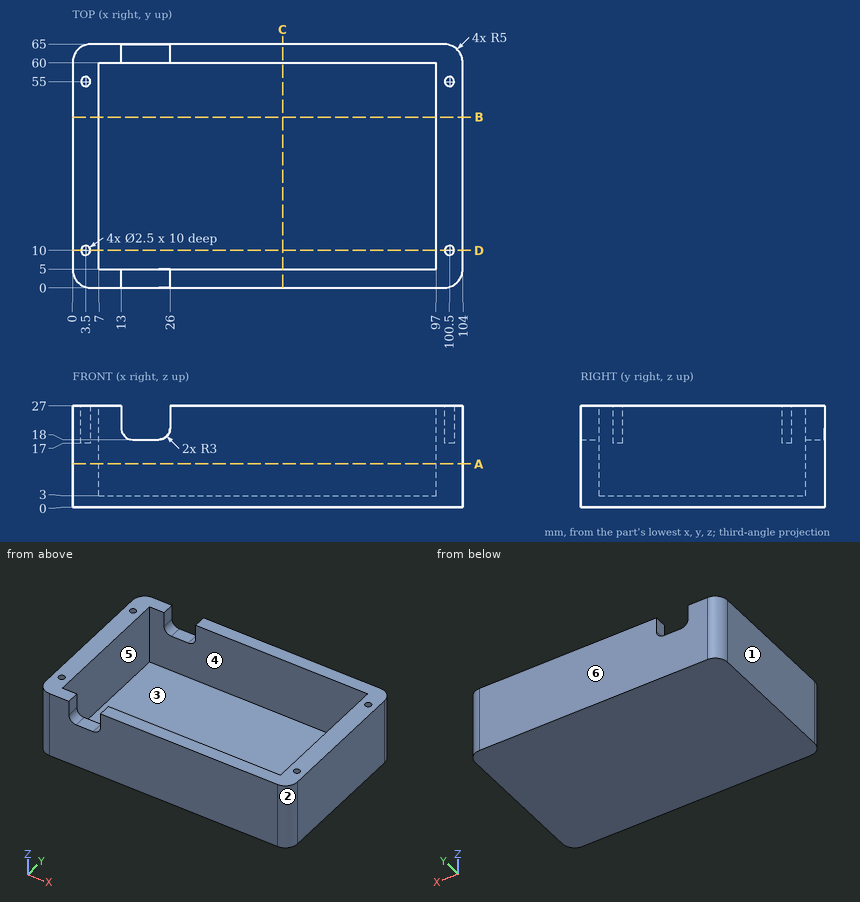
Study the drawing (mm; zero at the part's minimum x, y, z) and answer. A direction names the side the tool comes from. Round coordinates to 2 decimals unless told otherwise and drop trailing zeros. Write each loop counter-clockwise with the first axis right and the second up, starting at its lowest first coordinate (ties: lowest second). Pieces come first, ordered by that corner, then holes.
Q1. The mould has two halves that part along Y. Classify the marked faces 1, 2, 3 and 4: released by +Y, released by -Y, zero draft, split by the parting line, or undercut.
Values:
face 1: zero draft
face 2: released by -Y
face 3: undercut
face 4: undercut
Q2. Find section D-D on y = 10. Determine the outline of the cut face in (x, z).
Values:
outline: (0, 0) - (104, 0) - (104, 27) - (101.75, 27) - (101.75, 17) - (99.25, 17) - (99.25, 27) - (97, 27) - (97, 3) - (7, 3) - (7, 27) - (4.75, 27) - (4.75, 17) - (2.25, 17) - (2.25, 27) - (0, 27) - close
Q3. Flat-ended cylindrical pins translate along their axes: P1, Ø2, axis at x = 101, y = 54.5, coming from the +Z side; P2, Ø1.5, axis at y = 3, z = 23, coming from the +X side; P3, Ø2.5, axis at y = 62.5, z = 25, coming from the -X side; P4, Ø5, axis at x = 20.5, y = 51, coming from the +Z side. Find the tip coordinate at first contact, or state that the pin passes through.
Values:
P1: stops at z = 27
P2: stops at x = 103.84
P3: stops at x = 0.16
P4: stops at z = 3
Q4. Find section C-C on x = 56. Determine the outline of the cut face in (y, z).
Values:
outline: (0, 0) - (65, 0) - (65, 27) - (60, 27) - (60, 3) - (5, 3) - (5, 27) - (0, 27) - close
Q5. A tool of negligible diameter and unlimited length cuts with its end or side. For the marked faces 5 and 6, from which of +Z, -Z, +X, -X, +Y, -Y can it reach the whole face along a straight path? Write none if from no direction.
Values:
face 5: +Z
face 6: +Z, -Z, +X, -X, +Y
Q6. Find section B-B on y = 45.5. Determine the outline of the cut face in (x, z).
Values:
outline: (0, 0) - (104, 0) - (104, 27) - (97, 27) - (97, 3) - (7, 3) - (7, 27) - (0, 27) - close
Q7. Straight lines are drawn through the part: line 1 (Y direction, x = 30.5, z = 4.25); line 2 (X direction, y = 42, z = 13.75); line 3 (Y direction, x = 100.5, z = 24). For each, find the intervals that lie inside material, in ascending order.
Values:
line 1: y = 0 to 5, 60 to 65
line 2: x = 0 to 7, 97 to 104
line 3: y = 0.23 to 8.75, 11.25 to 53.75, 56.25 to 64.77
Q8. Find section A-A on z = 11.5. Determine the outline of the cut face in (x, y), and give its area (3 significant figures).
Values:
outline: (0, 5) arc R5 ccw to (5, 0) - (99, 0) arc R5 ccw to (104, 5) - (104, 60) arc R5 ccw to (99, 65) - (5, 65) arc R5 ccw to (0, 60) - close; hole (7, 5) - (97, 5) - (97, 60) - (7, 60) - close
area: 1,790 mm2
